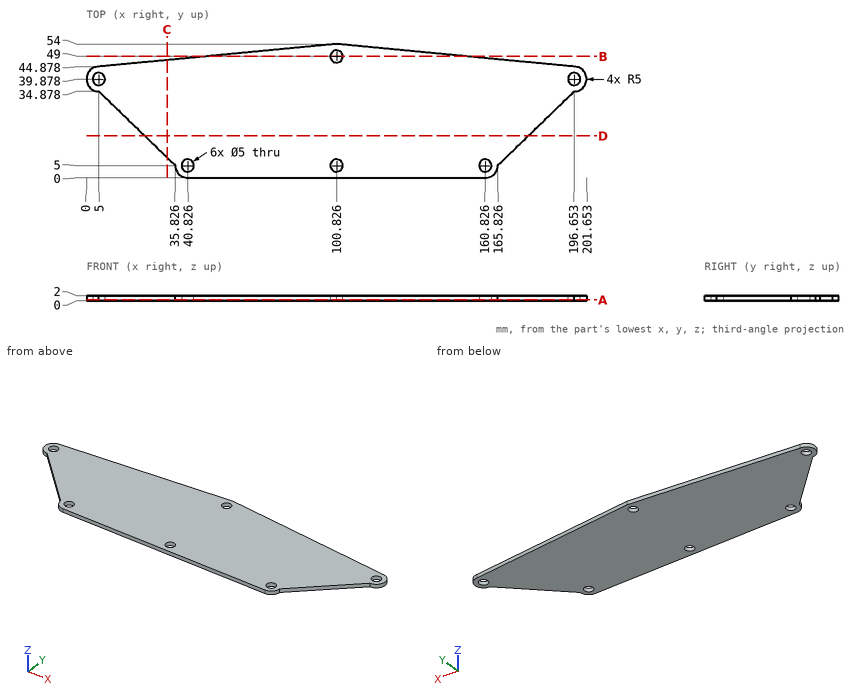
Print and shaded views of the part. All mm, measured from the part's lowest x, y and z. Coordinates: 2 decimals unless noted, no trailing zeros. Order: outer loops, then holes, each group sorted by start corner. A loop starts at its lowest first (then second) coordinate and runs counter-clockwise, first axis right, second up. Notation, with made-up numbers: M 23.25,47.25 L 50.25,47.25 A11 cw 50.25,60.25 Z; hole C 1,72 d1. An arc over 180 degrees is marked long. One line per question, with ' | ' between items. Start each with the question number.
Q1. Saw through at C-C (x = 32.5). List the corners of the cut face in (y, z).
Q2. Saw through at A-A (z = 0.4). List the corners of the cut face in (x, y).
Q3. Flat gauge pins, fed straight in: pin 1 Ø3 at (x, y) = (40.83, 5) entering from -Z; pin 2 Ø6 at (x, y) = (100.83, 49) entering from -Z. Where does each tip first touch, or does it go through?
Q4. Probe L1, parallel to Y at x = 5, z = 1; L2, parallel to X at y = 6, z = 1.65 (1 decimal); L3, parallel to Y at x = 99, z = 0.1 (1 decimal). List the from-to ranges inside material, lowest first. Write a range as from..to.
Q5. Saw through at D-D (y = 17). List the corners of the cut face in (x, z) (1 decimal).
Q6. Saw through at B-B (y = 49). List the corners of the cut face in (x, z), then the cut area to 3 significant figures.
Check values:
1) outline: M 8.22,0 L 47.5,0 L 47.5,2 L 8.22,2 Z
2) outline: M 5,34.88 L 35.83,5 A5 ccw 40.83,0 L 160.83,0 A5 ccw 165.83,5 L 196.65,34.88 A5 ccw 196.65,44.88 L 100.83,54 L 5,44.88 A5 ccw Z; hole C 5,39.88 d5; hole C 40.83,5 d5; hole C 100.83,5 d5; hole C 100.83,49 d5; hole C 160.83,5 d5; hole C 196.65,39.88 d5
3) pin 1: passes through | pin 2: stops at z = 0
4) L1: y = 34.88..37.38, 42.38..44.88 | L2: x = 34.8..38.5, 43.1..98.5, 103.1..158.5, 163.1..166.9 | L3: y = 0..3.3, 6.7..47.3, 50.7..53.8
5) outline: M 23.4,0 L 178.2,0 L 178.2,2 L 23.4,2 Z
6) outline: M 48.3,0 L 98.33,0 L 98.33,2 L 48.3,2 Z; M 103.33,0 L 153.35,0 L 153.35,2 L 103.33,2 Z | area: 200 mm2
